Geometry check sheet. Reference: the model listing, model coordinates, mm. A direction names the side the tool comes from. Give positions to 0.01 mm unless a question says otherwise; leave off trailing zeros. Order: outer loops, then holes, each group sorted by start corner. A loop starts at its lowest first (then second) coordinate and runs counter-clockwise, first axis right, second up. Notation, with made-up numbers: M 51,53.5 L 63,53.5 A18 cw 63,69.5 Z; hole C -36.5,44 d10. An arc over 180 degrees is marked long. Answer as a JSON object with one key per item and string values. Group by question number.
from build123d import *

# Parameters (mm, degrees)
F0_W     = 152.4
F0_H     = 114.3
F1_DEPTH = 152.4
F2_W     = 50.8
F2_H     = 76.2
F3_DEPTH = 114.3
F4_DEPTH = 114.3


with BuildPart() as f1:
    # F0 (on Front) → F1 (new body)
    with BuildSketch(Plane.XZ):
        Rectangle(F0_W, F0_H)
    extrude(amount=F1_DEPTH)

    # F2 (on face) → F3 (cut)
    with BuildSketch(Plane.XZ.offset(152.4)):
        with Locations((-50.8, 19.05)):
            Rectangle(F2_W, F2_H)
    extrude(amount=-F3_DEPTH, mode=Mode.SUBTRACT)

    # F2 (on face) → F4 (cut)
    with BuildSketch(Plane.XZ.offset(152.4)):
        with Locations((50.8, 19.05)):
            Rectangle(F2_W, F2_H)
    extrude(amount=-F4_DEPTH, mode=Mode.SUBTRACT)


solid = f1.part
1. Cross-section at C-C (x = 58). Record the cut outline in (y, z), and give its area (3 significant figures).
2. Access from +Z, -Z, +X, -X, +Y, -Y to the whole of each face (thin tool, end or side, straight path). Record for faces 1 (the flat face through (-51, -96, -19.05)), 2 (the flat face through (25.4, -96, 19)), 3 (the flat face through (-76.2, -58, -26)).
3. Cross-section at B-B (y = -136). Record the cut outline in (x, z).
4. Cross-section at A-A (z = 34.5). Record the cut outline in (x, y), and give its area (3 significant figures).
5. Thickness scan on line 1 along Y through (x, z) = (57.5, 51.5); line 2 along X through (y, z) = (-134.5, 14); line 3 along Z through (x, y) = (-30, -108.5). Record the ranges inside material, lowest first. Write a range as [from, to].
6. Depth check by flat-ended pin: pin 1 (4 mm diameter, centred on x = -50.5, y = -52, fed in from +Z); pin 2 (23 mm diameter, centred on y = -74.5, z = 38, fed in from -X). Enter the tip coordinate at first touch or a pass-through.
Report:
{
 "1": {"outline": "M -152.4,-57.15 L 0,-57.15 L 0,57.15 L -38.1,57.15 L -38.1,-19.05 L -152.4,-19.05 Z", "area": "8,710 mm2"},
 "2": {"face 1": "+Z, -X, -Y", "face 2": "+Z, +X, -Y", "face 3": "+Z, -Z, -X, +Y, -Y"},
 "3": {"outline": "M -76.2,-57.15 L 76.2,-57.15 L 76.2,-19.05 L 25.4,-19.05 L 25.4,57.15 L -25.4,57.15 L -25.4,-19.05 L -76.2,-19.05 Z"},
 "4": {"outline": "M -76.2,-38.1 L -25.4,-38.1 L -25.4,-152.4 L 25.4,-152.4 L 25.4,-38.1 L 76.2,-38.1 L 76.2,0 L -76.2,0 Z", "area": "11,600 mm2"},
 "5": {"line 1": "y = [-38.1, 0]", "line 2": "x = [-25.4, 25.4]", "line 3": "z = [-57.15, -19.05]"},
 "6": {"pin 1": "stops at z = -19.05", "pin 2": "stops at x = -25.4"}
}
